The model under review builds one solid part; all positions refer to its coordinate system, in mm. A direction names the side the tool comes from. Round coordinates to 2 decimals unless told otherwise and drop trailing zeros. Loops run counter-clockwise (first coordinate to the right, second up) from the corner with the lowest first, then second, coordinate; pieces in that order, holes last. Notation, with made-up numbers: M 50,-14 L 60,-14 A20 cw 60,12 Z; hole C 46,-36.75 d9. An arc over 180 degrees is marked long. Return JSON: item names as keys, results as strings. Group by question number.
Q1. For faces 1 (the face through (5, -218.25, 33)), 2 (the face through (-12, -226.5, 44)), 3 (the face through (-4, -32, 44)), 4 (the face through (-7, -222.5, 44)), list the 3-axis set-ups (+Z, -Z, +X, -X, +Y, -Y) from which the entire face can be reached by the end or side of a thin tool; tool diameter is ignored.
Q2. To check wall thickness, follow line 1 along X through (y, z) = (-107.5, 40); line 2 along Y through (x, z) = (220, 46.5); line 3 along X through (y, z) = (-224.5, 72). State the ranges of each line that lie inside material, in increasing order.
Q3. Consider section A-A (z = 7.5). State the section outline as (x, y) points, and give its area (3 significant figures).
Q4. Clearance check with flat-ended pins moving along their axes: pin 1 Ø17.5 at (y, z) = (-255, 54.5) entering from -X; pin 2 Ø3 at (x, y) = (2.5, -127.5) entering from +Z; pin 3 Ø12 at (x, z) = (-11, 56) entering from +Y. State where each tip first meets the part, or that it passes through.
Q5. Consider section D-D (y = 23). State the section outline as (x, z) points.
Q6. Consider section B-B (y = -184). State the section outline as (x, z) points, and give its area (3 significant figures).
Q7. Consider section C-C (x = 241.5). State the section outline as (y, z) points.
Q8. Draft analysis for pull direction X (two halves, no side actions). For faces 5 (the face through (130, 3, 90)), 6 (the face through (375.5, -87, 44)), 7 (the face through (311, -225, 45)), state which applies: pulls with the +X half, pulls with the -X half, needs draft (parallel to the pull), parting line crosses it, or undercut.
from build123d import *

# Parameters (mm, degrees)
F1_DEPTH = 90
F2_DEPTH = 1
F0_W     = 10.5
F0_H     = 140.5
F3_DEPTH = 66
F4_W     = 157
F4_H     = 14.86842
F5_DEPTH = 4


with BuildPart() as f1:
    # F0 (on Top) → F1 (new body)
    with BuildSketch(Plane.XY):
        Polygon((0, -73.5), (0, 0), (275.5, 0), (275.5, 59), (271.5, 59), (271.5, 4), (-4, 4), (-4, -69.5), (-19, -69.5), (-19, -226.5), (-4, -226.5), (-4, -284.5), (253, -284.5), (253, -229), (375.5, -229), (375.5, 59), (371.5, 59), (371.5, 0), (371.5, -225), (249, -225), (249, -280.5), (0, -280.5), (0, -222.5), (-15, -222.5), (-15, -73.5), align=None)
    extrude(amount=F1_DEPTH)

    # F0 (on Top) → F2 (join)
    with BuildSketch(Plane.XY):
        Polygon((275.5, 0), (0, 0), (0, -73.5), (0, -77.75), (10.5, -77.75), (10.5, -218.25), (0, -218.25), (0, -222.5), (0, -280.5), (249, -280.5), (249, -225), (371.5, -225), (371.5, 0), (371.5, 59), (275.5, 59), align=None)
    extrude(amount=F2_DEPTH)

    # F0 (on Top) → F3 (join)
    with BuildSketch(Plane.XY):
        with Locations((5.25, -148)):
            Rectangle(F0_W, F0_H)
    extrude(amount=F3_DEPTH)

    # F4 (on face) → F5 (cut)
    with BuildSketch(Plane(origin=(-19, 0, 0), x_dir=(0, -1, 0), z_dir=(-1, 0, 0))):
        with Locations((148, 82.56579)):
            Rectangle(F4_W, F4_H)
    extrude(amount=-F5_DEPTH, mode=Mode.SUBTRACT)


solid = f1.part
Values:
{
 "1": {"face 1": "+Z", "face 2": "+Z, -Z, -X, -Y", "face 3": "+Z, -Z, -X, +Y", "face 4": "+Z, -Z"},
 "2": {"line 1": "x = -19 to -15, 0 to 10.5, 371.5 to 375.5", "line 2": "y = -284.5 to -280.5, 0 to 4", "line 3": "x = -19 to 0, 371.5 to 375.5"},
 "3": {"outline": "M -19,-226.5 L -4,-226.5 L -4,-284.5 L 253,-284.5 L 253,-229 L 375.5,-229 L 375.5,59 L 371.5,59 L 371.5,-225 L 249,-225 L 249,-280.5 L 0,-280.5 L 0,-222.5 L -15,-222.5 L -15,-73.5 L 0,-73.5 L 0,0 L 275.5,0 L 275.5,59 L 271.5,59 L 271.5,4 L -4,4 L -4,-69.5 L -19,-69.5 Z; M 0,-218.25 L 10.5,-218.25 L 10.5,-77.75 L 0,-77.75 Z", "area": "6,930 mm2"},
 "4": {"pin 1": "stops at x = -4", "pin 2": "stops at z = 66", "pin 3": "stops at y = -69.5"},
 "5": {"outline": "M 271.5,0 L 375.5,0 L 375.5,90 L 371.5,90 L 371.5,1 L 275.5,1 L 275.5,90 L 271.5,90 Z"},
 "6": {"outline": "M -19,0 L -15,0 L -15,75.13 L -19,75.13 Z; M 0,0 L 375.5,0 L 375.5,90 L 371.5,90 L 371.5,1 L 10.5,1 L 10.5,66 L 0,66 Z", "area": "1,710 mm2"},
 "7": {"outline": "M -284.5,0 L 4,0 L 4,90 L 0,90 L 0,1 L -280.5,1 L -280.5,90 L -284.5,90 Z"},
 "8": {"face 5": "needs draft", "face 6": "pulls with the +X half", "face 7": "undercut"}
}
